Build history of the part. All positions in model axes, mm. Face numbers are marked on the shaded views. A direction names the side the tool comes from. Give positions to 0.01 mm unless a question says otherwise; leave off trailing zeros. Loops run counter-clockwise (first coordinate to the right, second up) from the corner with the lowest first, then second, coordinate; pieces in that order, holes last. Notation, with made-up numbers: (-3, 47) -> (54, 47) arc R18 ccw to (54, 78) -> close; hole circle Ø10 at (10.25, -26). An arc over 180 degrees is marked (long way). Answer as a JSON object with one key per item and string values. Group by question number.
from build123d import *

# Parameters (mm, degrees)
F0_W     = 25
F0_H     = 25
F0_R     = 2
F0_W_2   = 15.5
F0_H_2   = 15.5
F1_DEPTH = 25
F2_W     = 15.5
F2_H     = 15.5
F3_DEPTH = 25
F4_W     = 15.5
F4_H     = 15.5
F5_DEPTH = 25
F6_DEPTH = 25
F8_SIZE  = 3
F7_R     = 2
F9_DEPTH = 25


with BuildPart() as f1:
    # F0 (on Top) → F1 (new body)
    with BuildSketch(Plane.XY):
        with Locations((-47.5, 37.5)):
            Rectangle(F0_W, F0_H)
        with Locations((-47.5, 37.5)):
            Circle(F0_R, mode=Mode.SUBTRACT)
        with Locations((-22.5, 12.5)):
            Rectangle(F0_W, F0_H)
        with Locations((-22.5, 12.5)):
            Circle(F0_R, mode=Mode.SUBTRACT)
        with Locations((-47.5, 12.5)):
            Rectangle(F0_W, F0_H)
        with Locations((-47.5, 12.5)):
            Rectangle(F0_W_2, F0_H_2, mode=Mode.SUBTRACT)
        with Locations((-47.5, 12.5)):
            Rectangle(F0_W_2, F0_H_2)
    extrude(amount=-F1_DEPTH)

    # F2 (on face) → F3 (cut)
    with BuildSketch(Plane.YZ.offset(-10)):
        with Locations((12.5, -12.5)):
            Rectangle(F2_W, F2_H)
    extrude(amount=-F3_DEPTH, mode=Mode.SUBTRACT)

    # F4 (on face) → F5 (cut)
    with BuildSketch(Plane(origin=(0, 50, 0), x_dir=(-1, 0, 0), z_dir=(0, 1, 0))):
        with Locations((47.5, -12.5)):
            Rectangle(F4_W, F4_H)
    extrude(amount=-F5_DEPTH, mode=Mode.SUBTRACT)

    # F0 (on Top) → F6 (join)
    with BuildSketch(Plane.XY):
        with Locations((-47.5, 12.5)):
            Rectangle(F0_W, F0_H)
        with Locations((-47.5, 12.5)):
            Rectangle(F0_W_2, F0_H_2, mode=Mode.SUBTRACT)
    extrude(amount=F6_DEPTH)

    # F8
    f8_edges = [f1.edges().sort_by_distance(p)[0] for p in [
        (-60, 0, 0),
        (-35, 0, -25),
        (-60, 25, -25),
        (-35, 0, 12.5),
        (-22.5, 0, 0),
        (-35, 37.5, -25),
        (-22.5, 25, -25),
        (-60, 37.5, 0),
        (-60, 25, 12.5),
    ]]
    chamfer(f8_edges, length=F8_SIZE)

    # F7 (on face) → F9 (cut)
    with BuildSketch(Plane.YZ.offset(-35)):
        with Locations((12.5, 12.5)):
            Circle(F7_R)
    extrude(amount=-F9_DEPTH, mode=Mode.SUBTRACT)


solid = f1.part
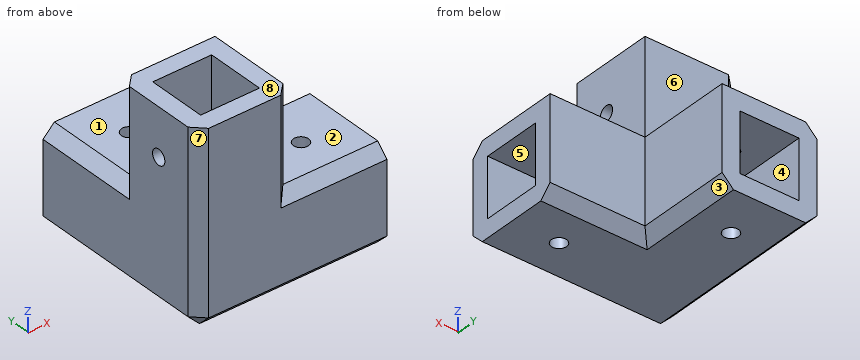
(1) 3-axis set-ups, long thin cutter, end or side, ignore diameter. For the marked faces 1, 2, 3 and 4: which of +Z, -Z, +X, -X, +Y, -Y reach the whole face in a straight line?
(2) Pull direction Y, two halves, no side cores. Call the marked faces 5, 6, 7 and 8: pulls with the +Y half, pulls with the -Y half, needs draft (parallel to the pull), parting line crosses it, or undercut.
(3) Saw through at B-B on x = -47.5. List the corners of the cut face in (y, z), plus the area to 3 significant figures.
(4) Saw through at D-D on y = 43. List the corners of the cut face in (x, z), plus the area to 3 significant figures.
(5) Saw through at A-A on y = 37.5. List the corners of the cut face in (x, z).
(6) Saw through at C-C on z = 12.5. List the corners of the cut face in (x, y), plus the area to 3 significant figures.
(7) Probe line 1 along X through (y, z) = (9, 16.5); line 2 along Y through (x, z) = (-15, -11.5); line 3 along Z through (x, y) = (-47, 29). List the from-to ranges inside material, lowest first. Write a range as [from, to].
(8) Pin check, flat tips, straight feed: pin 1 (4.5 mm diameter, centred on y = 10, z = -12.5, fed in from +X); pin 2 (12.5 mm diameter, centred on x = -49, z = 16.5, fed in from +Y); pin 3 (5 mm diameter, centred on y = 12.5, z = 12.5, fed in from -X); pin 4 (12.5 mm diameter, centred on x = -20.5, y = 13, fed in from +Z). Stop position of each tip, or through.
Calculated:
{
 "1": {"face 1": "+Z, +X, -X, +Y", "face 2": "+Z, +X, +Y, -Y", "face 3": "-Z, +X, +Y", "face 4": "+Y"},
 "2": {"face 5": "undercut", "face 6": "pulls with the +Y half", "face 7": "pulls with the -Y half", "face 8": "needs draft"},
 "3": {"outline": "(0, -22) -> (3, -25) -> (35.5, -25) -> (35.5, -20.25) -> (25, -20.25) -> (25, -4.75) -> (35.5, -4.75) -> (35.5, 0) -> (25, 0) -> (25, 25) -> (20.25, 25) -> (20.25, 0) -> (4.75, 0) -> (4.75, 25) -> (0, 25) -> close; (39.5, -25) -> (50, -25) -> (50, -20.25) -> (39.5, -20.25) -> close; (39.5, -4.75) -> (50, -4.75) -> (50, 0) -> (39.5, 0) -> close", "area": "1,060 mm^2"},
 "4": {"outline": "(-60, -22) -> (-57, -25) -> (-38, -25) -> (-35, -22) -> (-35, 0) -> (-57, 0) -> (-60, -3) -> close; hole (-55.25, -20.25) -> (-39.75, -20.25) -> (-39.75, -4.75) -> (-55.25, -4.75) -> close", "area": "371 mm^2"},
 "5": {"outline": "(-60, -22) -> (-57, -25) -> (-49.5, -25) -> (-49.5, -20.25) -> (-55.25, -20.25) -> (-55.25, -4.75) -> (-49.5, -4.75) -> (-49.5, 0) -> (-57, 0) -> (-60, -3) -> close; (-45.5, -25) -> (-38, -25) -> (-35, -22) -> (-35, 0) -> (-45.5, 0) -> (-45.5, -4.75) -> (-39.75, -4.75) -> (-39.75, -20.25) -> (-45.5, -20.25) -> close"},
 "6": {"outline": "(-60, 3) -> (-57, 0) -> (-38, 0) -> (-35, 3) -> (-35, 10.5) -> (-39.75, 10.5) -> (-39.75, 4.75) -> (-55.25, 4.75) -> (-55.25, 10.5) -> (-60, 10.5) -> close; (-60, 14.5) -> (-55.25, 14.5) -> (-55.25, 20.25) -> (-39.75, 20.25) -> (-39.75, 14.5) -> (-35, 14.5) -> (-35, 25) -> (-57, 25) -> (-60, 22) -> close", "area": "333 mm^2"},
 "7": {"line 1": "x = [-60, -55.25], [-39.75, -35]", "line 2": "y = [0, 4.75], [20.25, 25]", "line 3": "z = [-25, -20.25], [-4.75, 0]"},
 "8": {"pin 1": "stops at x = -35", "pin 2": "stops at y = 25", "pin 3": "stops at x = -60", "pin 4": "stops at z = 0"}
}
